```python
from build123d import *

# Parameters (mm, degrees)
SKETCH1_R           = 63.5
SKETCH1_R_2         = 1.4224
SKETCH1_R_3         = 4
SKETCH1_R_4         = 3.55
SKETCH1_R_5         = 1.397
SKETCH1_W           = 0.5334
SKETCH1_H           = 0.5334
SKETCH1_W_2         = 3.175
SKETCH1_H_2         = 19.05
SKETCH1_W_3         = 25.556343598
SKETCH1_H_3         = 3.175
SKETCH1_W_4         = 25.4
BOSS_EXTRUDE1_DEPTH = 3.175


with BuildPart() as part:
    # Sketch1 → Boss-Extrude1 (new body)
    with BuildSketch(Plane.XY):
        with BuildLine():
            Line((-88.9, 0), (-88.9, -152.4))
            Line((-88.9, -152.4), (88.9, -152.4))
            Line((88.9, -152.4), (88.9, 0))
            ThreePointArc((88.9, 0), (0, 88.9), (-88.9, 0))
        make_face()
        Circle(SKETCH1_R, mode=Mode.SUBTRACT)
        with Locations((-84.1375, -100.33)):
            Circle(SKETCH1_R_2, mode=Mode.SUBTRACT)
        with Locations((84.1375, -100.33)):
            Circle(SKETCH1_R_2, mode=Mode.SUBTRACT)
        with Locations((22.225, -107.95)):
            Circle(SKETCH1_R_3, mode=Mode.SUBTRACT)
        with Locations((44.45, -107.95)):
            Circle(SKETCH1_R_4, mode=Mode.SUBTRACT)
        with Locations((66.675, -107.95)):
            Circle(SKETCH1_R_4, mode=Mode.SUBTRACT)
        with Locations((-15.977581987, -96.52)):
            Circle(SKETCH1_R_5, mode=Mode.SUBTRACT)
        with Locations((-46.457581987, -129.54)):
            Circle(SKETCH1_R_5, mode=Mode.SUBTRACT)
        with Locations((-1.30175, 69.85)):
            Rectangle(SKETCH1_W, SKETCH1_H, mode=Mode.SUBTRACT)
        with Locations((1.30175, 69.85)):
            Rectangle(SKETCH1_W, SKETCH1_H, mode=Mode.SUBTRACT)
        Polygon((33.700032455, 61.50706843), (34.161970406, 61.24036843), (33.895270406, 60.778430479), (33.433332455, 61.045130479), align=None, mode=Mode.SUBTRACT)
        Polygon((35.954729594, 60.20531843), (35.688029594, 59.743380479), (36.149967545, 59.476680479), (36.416667545, 59.93861843), align=None, mode=Mode.SUBTRACT)
        Polygon((59.93861843, 36.416667545), (60.20531843, 35.954729594), (59.743380479, 35.688029594), (59.476680479, 36.149967545), align=None, mode=Mode.SUBTRACT)
        Polygon((61.24036843, 34.161970406), (60.778430479, 33.895270406), (61.045130479, 33.433332455), (61.50706843, 33.700032455), align=None, mode=Mode.SUBTRACT)
        with Locations((69.85, 1.30175)):
            Rectangle(SKETCH1_W, SKETCH1_H, mode=Mode.SUBTRACT)
        with Locations((69.85, -1.30175)):
            Rectangle(SKETCH1_W, SKETCH1_H, mode=Mode.SUBTRACT)
        Polygon((61.50706843, -33.700032455), (61.24036843, -34.161970406), (60.778430479, -33.895270406), (61.045130479, -33.433332455), align=None, mode=Mode.SUBTRACT)
        Polygon((60.20531843, -35.954729594), (59.743380479, -35.688029594), (59.476680479, -36.149967545), (59.93861843, -36.416667545), align=None, mode=Mode.SUBTRACT)
        Polygon((36.416667545, -59.93861843), (35.954729594, -60.20531843), (35.688029594, -59.743380479), (36.149967545, -59.476680479), align=None, mode=Mode.SUBTRACT)
        Polygon((34.161970406, -61.24036843), (33.895270406, -60.778430479), (33.433332455, -61.045130479), (33.700032455, -61.50706843), align=None, mode=Mode.SUBTRACT)
        with Locations((1.30175, -69.85)):
            Rectangle(SKETCH1_W, SKETCH1_H, mode=Mode.SUBTRACT)
        with Locations((-1.30175, -69.85)):
            Rectangle(SKETCH1_W, SKETCH1_H, mode=Mode.SUBTRACT)
        Polygon((-33.700032455, -61.50706843), (-34.161970406, -61.24036843), (-33.895270406, -60.778430479), (-33.433332455, -61.045130479), align=None, mode=Mode.SUBTRACT)
        Polygon((-35.954729594, -60.20531843), (-35.688029594, -59.743380479), (-36.149967545, -59.476680479), (-36.416667545, -59.93861843), align=None, mode=Mode.SUBTRACT)
        Polygon((-59.93861843, -36.416667545), (-60.20531843, -35.954729594), (-59.743380479, -35.688029594), (-59.476680479, -36.149967545), align=None, mode=Mode.SUBTRACT)
        Polygon((-61.24036843, -34.161970406), (-60.778430479, -33.895270406), (-61.045130479, -33.433332455), (-61.50706843, -33.700032455), align=None, mode=Mode.SUBTRACT)
        with Locations((-69.85, -1.30175)):
            Rectangle(SKETCH1_W, SKETCH1_H, mode=Mode.SUBTRACT)
        with Locations((-69.85, 1.30175)):
            Rectangle(SKETCH1_W, SKETCH1_H, mode=Mode.SUBTRACT)
        Polygon((-61.50706843, 33.700032455), (-61.24036843, 34.161970406), (-60.778430479, 33.895270406), (-61.045130479, 33.433332455), align=None, mode=Mode.SUBTRACT)
        Polygon((-60.20531843, 35.954729594), (-59.743380479, 35.688029594), (-59.476680479, 36.149967545), (-59.93861843, 36.416667545), align=None, mode=Mode.SUBTRACT)
        Polygon((-36.416667545, 59.93861843), (-35.954729594, 60.20531843), (-35.688029594, 59.743380479), (-36.149967545, 59.476680479), align=None, mode=Mode.SUBTRACT)
        Polygon((-34.161970406, 61.24036843), (-33.895270406, 60.778430479), (-33.433332455, 61.045130479), (-33.700032455, 61.50706843), align=None, mode=Mode.SUBTRACT)
        with Locations((-77.7875, 22.20976)):
            Rectangle(SKETCH1_W_2, SKETCH1_H_2, mode=Mode.SUBTRACT)
        with Locations((-77.7875, -73.04024)):
            Rectangle(SKETCH1_W_2, SKETCH1_H_2, mode=Mode.SUBTRACT)
        with Locations((-84.1375, -140.335)):
            Rectangle(SKETCH1_W_2, SKETCH1_H_2, mode=Mode.SUBTRACT)
        with Locations((-84.1375, -60.325)):
            Rectangle(SKETCH1_W_2, SKETCH1_H_2, mode=Mode.SUBTRACT)
        with Locations((84.1375, -140.335)):
            Rectangle(SKETCH1_W_2, SKETCH1_H_2, mode=Mode.SUBTRACT)
        with Locations((77.7875, 22.20976)):
            Rectangle(SKETCH1_W_2, SKETCH1_H_2, mode=Mode.SUBTRACT)
        with Locations((84.1375, -60.325)):
            Rectangle(SKETCH1_W_2, SKETCH1_H_2, mode=Mode.SUBTRACT)
        with Locations((77.7875, -73.04024)):
            Rectangle(SKETCH1_W_2, SKETCH1_H_2, mode=Mode.SUBTRACT)
        with Locations((-0.078171799, 80.9625)):
            Rectangle(SKETCH1_W_3, SKETCH1_H_3, mode=Mode.SUBTRACT)
        with Locations((0, -80.9625)):
            Rectangle(SKETCH1_W_4, SKETCH1_H_3, mode=Mode.SUBTRACT)
    extrude(amount=BOSS_EXTRUDE1_DEPTH)


solid = part.part
```
Source: CAD feature listing. Evaluate the final solid. Frame: model axes, mm. Give positions to 0.01 mm unless a question says otherwise; leave off trailing zeros. Loops run counter-clockwise (first coordinate to the right, second up) from the corner with the lowest first, then second, coordinate; pieces in that order, holes last. Notation, with made-up numbers: (54, 47) -> (80, 47) arc R34 ccw to (80, 82) -> close; hole circle Ø5 at (56, 76). An arc over 180 degrees is marked (long way). Use a Markdown table: item, result. Add a question column.
(1) Section query A-A (y = -107.95). Output: boundary loops of the cut face in (x, z) (3 decimals).
(2) First-contact query: pin 1 Ø0.6 at (x, z) = (-1.5, 2) entering from +Y; pin 2 Ø0.6 at (y, z) = (70, 2) entering from +X. Flat tips, straight axial feed; report the tip coordinate or a pass-through.
(3) Section query B-B (x = -20). Output: boundary loops of the cut face in (y, z) (3 decimals).
(4) Pull-direction query (X, two-part tool) for faces 1 (the face through (46.09, -111.1, 1.57)), 2 (the face through (-1, -84, 3.175)), 3 (the face through (1.95, 88.88, 1.57)); classes: +X half, -X half, draft (parallel to the pull), parting line (faces both ways), or undercut.
(5) Ray query, line 1 (X direction, y = -100.33, z = 1.4); line 2 (X direction, y = -135.5, z = 1.15) (3 decimals); line 3 (Y direction, x = 0, z = 1.15) (3 decimals). Return the intervals inside material, ascending.
(6) Section query D-D (x = 44.45). Output: boundary loops of the cut face in (y, z) (3 decimals).
(7) Section query C-C (y = -137). Output: boundary loops of the cut face in (x, z) (3 decimals).
Checked values:
| question | item | result |
|---|---|---|
| 1 | outline | (-88.9, 0) -> (18.225, 0) -> (18.225, 3.175) -> (-88.9, 3.175) -> close; (26.225, 0) -> (40.9, 0) -> (40.9, 3.175) -> (26.225, 3.175) -> close; (48, 0) -> (63.125, 0) -> (63.125, 3.175) -> (48, 3.175) -> close; (70.225, 0) -> (88.9, 0) -> (88.9, 3.175) -> (70.225, 3.175) -> close |
| 2 | pin 1 | y = 88.89 |
| 2 | pin 2 | x = 55.18 |
| 3 | outline | (-152.4, 0) -> (-60.268, 0) -> (-60.268, 3.175) -> (-152.4, 3.175) -> close; (60.268, 0) -> (86.621, 0) -> (86.621, 3.175) -> (60.268, 3.175) -> close |
| 4 | face 1 | undercut |
| 4 | face 2 | draft |
| 4 | face 3 | parting line |
| 5 | line 1 | -88.9 to -85.56, -82.72 to 82.72, 85.56 to 88.9 |
| 5 | line 2 | -88.9 to -85.725, -82.55 to 82.55, 85.725 to 88.9 |
| 5 | line 3 | -152.4 to -82.55, -79.375 to -63.5, 63.5 to 79.375, 82.55 to 88.9 |
| 6 | outline | (-152.4, 0) -> (-111.5, 0) -> (-111.5, 3.175) -> (-152.4, 3.175) -> close; (-104.4, 0) -> (-45.348, 0) -> (-45.348, 3.175) -> (-104.4, 3.175) -> close; (45.348, 0) -> (76.99, 0) -> (76.99, 3.175) -> (45.348, 3.175) -> close |
| 7 | outline | (-88.9, 0) -> (-85.725, 0) -> (-85.725, 3.175) -> (-88.9, 3.175) -> close; (-82.55, 0) -> (82.55, 0) -> (82.55, 3.175) -> (-82.55, 3.175) -> close; (85.725, 0) -> (88.9, 0) -> (88.9, 3.175) -> (85.725, 3.175) -> close |
